Geometry: final body of the model. Coordinates: model frame, mm. Face numbers are marked on the shaded views. A direction names the side the tool comes from. Give positions to 0.01 mm unless a question says otherwise; leave off trailing zeros. Write each loop counter-clockwise with the first axis right and the second up, starting at its lowest first coordinate (ties: lowest second). Pieces come first, ordered by that corner, then holes. Notation, with made-up numbers: M -39.75,-30 L -5.75,-30 A17 ccw -5.75,-2 Z; hole C 7.25,-29 d3. An arc over 180 degrees is marked long. Use one line per item in the form item = value. Start each with the question number.
Item 1: Access query for the marked faces 1 and 2. Directions: +Z, -Z, +X, -X, +Y, -Y. A direction counts if a zero-diameter tool reaches every point of the face in a straight line with its end or side. Return the directions, or none.
Item 2: Material intervals for line 1 along X through (y, z) = (-7.5, 1.05); line 2 along X through (y, z) = (-15.5, 2.2); line 3 along Y through (x, z) = (-57.5, 1.65), sorted ascending. Write a range as from..to.
Item 3: Section query A-A on y = 8. Return loops of the section in (x, z), then the cut area to 3 significant figures.
Item 4: Pull-direction query (Y, two-part tool) for the marked faces 3, 4 and 5; classes: released by +Y, released by -Y, zero draft, split by the parting line, or undercut.
Item 5: Section query B-B on x = -43. Return loops of the section in (y, z).
Item 6: Section query C-C on y = 1.5. Return loops of the section in (x, z), then the cut area to 3 significant figures.
Item 7: Contact query for a flat-ended pin moving along its axis: P1, Ø2, axis at x = -57.5, y = -7.5, coming from the +Z side. Output: stop coordinate, or through.
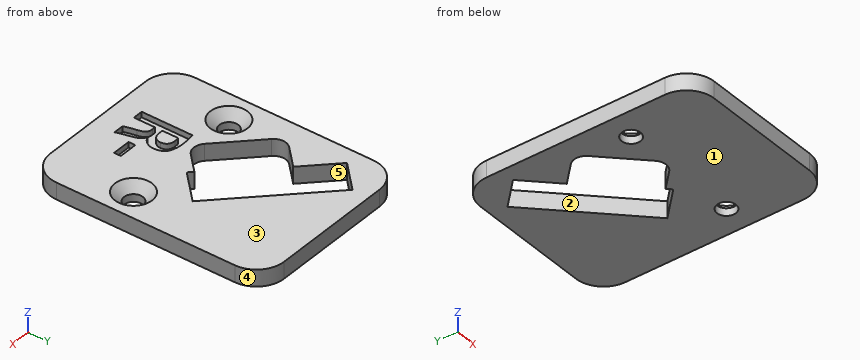
from build123d import *

# Parameters (mm, degrees)
SKETCH2_W                                           = 32
SKETCH2_H                                           = 42.204432033
BOSS_EXTRUDE2_DEPTH                                 = 3
FILLET1_R                                           = 5
SKETCH3_W                                           = 3.336226562
SKETCH3_H                                           = 1.222113554
CUT_EXTRUDE1_DEPTH                                  = 1
CSK_FOR_M3_COUNTERSUNK_FLAT_HEAD_SCREW1_D           = 3.4
CSK_FOR_M3_COUNTERSUNK_FLAT_HEAD_SCREW1_DEPTH       = 20
CSK_FOR_M3_COUNTERSUNK_FLAT_HEAD_SCREW1_CSINK_D     = 6.7
CSK_FOR_M3_COUNTERSUNK_FLAT_HEAD_SCREW1_CSINK_ANGLE = 90
CSK_FOR_M3_COUNTERSUNK_FLAT_HEAD_SCREW1_TIP         = 1.021463052
CUT_EXTRUDE3_DEPTH                                  = 10


with BuildPart() as part:
    # Sketch2 → Boss-Extrude2 (new body)
    with BuildSketch(Plane.XY):
        with Locations((-46.5, -1.397783984)):
            Rectangle(SKETCH2_W, SKETCH2_H)
    extrude(amount=BOSS_EXTRUDE2_DEPTH)

    # Fillet1
    fillet1_edges = [part.edges().sort_by_distance(p)[0] for p in [
        (-62.5, 19.704432033, 1.5),
        (-30.5, 19.704432033, 1.5),
        (-30.5, -22.5, 1.5),
        (-62.5, -22.5, 1.5),
    ]]
    fillet(fillet1_edges, radius=FILLET1_R)

    # Sketch3 → Cut-Extrude1 (cut)
    with BuildSketch(Plane.XY.offset(3)):
        with BuildLine():
            Line((-51.381425439, -18.458875061), (-49.597421385, -18.458875061))
            Line((-49.597421385, -18.458875061), (-49.597421385, -14.672122679))
            Line((-49.597421385, -14.672122679), (-48.991938415, -14.672122679))
            add(Edge.make_bspline(
                [(-48.991938415, -14.672122679), (-48.942050564, -14.6725211), (-48.843919084, -14.673304811), (-48.701136712, -14.687536776), (-48.566178681, -14.711269605), (-48.441222715, -14.74890661), (-48.32427753, -14.795186794), (-48.218202264, -14.856795477), (-48.11890245, -14.926037335), (-48.029787183, -15.010644116), (-47.94865002, -15.109304476), (-47.870329282, -15.22163632), (-47.801359571, -15.353586411), (-47.734046558, -15.500135947), (-47.675917518, -15.664809001), (-47.618382932, -15.843956856), (-47.570508607, -16.041536599), (-47.542007813, -16.179191645), (-47.527206071, -16.25068209)],
                knots=[0, 0, 0, 0, 0.000149599, 0.000294267, 0.000429961, 0.000559969, 0.000685182, 0.000806276, 0.000927115, 0.001047609, 0.001173509, 0.001309883, 0.001457588, 0.001619475, 0.001793345, 0.001981055, 0.002183769, 0.002402801, 0.002402801, 0.002402801, 0.002402801], degree=3))
            add(Edge.make_bspline(
                [(-47.527206071, -16.25068209), (-47.500027556, -16.387123246), (-47.447932519, -16.648649934), (-47.367799698, -17.023584407), (-47.286395279, -17.362673147), (-47.211369572, -17.666100231), (-47.134583702, -17.927379781), (-47.069987521, -18.146751884), (-47.009849282, -18.32008565), (-46.966417008, -18.417682148), (-46.947756493, -18.45961412)],
                knots=[0, 0, 0, 0, 0.000417367, 0.000799998, 0.001150089, 0.001463532, 0.001737527, 0.001966934, 0.002149658, 0.002287303, 0.002287303, 0.002287303, 0.002287303], degree=3))
            Line((-46.947756493, -18.45961412), (-45.111733669, -18.458875061))
            add(Edge.make_bspline(
                [(-45.111733669, -18.458875061), (-45.136394395, -18.402686862), (-45.192836553, -18.274086301), (-45.264632108, -18.048232695), (-45.345858267, -17.770288113), (-45.428958388, -17.444111213), (-45.51591734, -17.08294144), (-45.610026609, -16.699954349), (-45.704155867, -16.299301278), (-45.768362179, -16.026508782), (-45.80114869, -15.887209172)],
                knots=[0, 0, 0, 0, 0.000183977, 0.000421076, 0.000710029, 0.001052867, 0.00143062, 0.001824558, 0.002235981, 0.002665299, 0.002665299, 0.002665299, 0.002665299], degree=3))
            add(Edge.make_bspline(
                [(-45.80114869, -15.887209172), (-45.828641018, -15.773168942), (-45.881780404, -15.5527428), (-45.987295673, -15.242137194), (-46.108403792, -14.961961493), (-46.246109756, -14.712628496), (-46.405457942, -14.494327391), (-46.588613385, -14.309294243), (-46.799272936, -14.160659908), (-46.954100619, -14.089741414), (-47.032040068, -14.054041414)],
                knots=[0, 0, 0, 0, 0.000351778, 0.000679945, 0.00098268, 0.001266475, 0.001532679, 0.001790935, 0.002044255, 0.002301038, 0.002301038, 0.002301038, 0.002301038], degree=3))
            Line((-47.032040068, -14.054041414), (-47.030656262, -14.017001018))
            add(Edge.make_bspline(
                [(-47.030656262, -14.017001018), (-46.922273974, -13.970005767), (-46.706005829, -13.876230519), (-46.411856808, -13.676157256), (-46.14181559, -13.438863882), (-45.942211161, -13.208200023), (-45.802357006, -13.003332314), (-45.709339658, -12.840203194), (-45.629535439, -12.668874791), (-45.565066724, -12.488727388), (-45.51180506, -12.300576236), (-45.473637881, -12.103222096), (-45.448546386, -11.89781805), (-45.443663093, -11.757970901), (-45.441187588, -11.68707768)],
                knots=[0, 0, 0, 0, 0.000353722, 0.000705825, 0.001061629, 0.00143016, 0.001617179, 0.001805135, 0.001992894, 0.002183416, 0.002378543, 0.002578963, 0.00278587, 0.002998596, 0.002998596, 0.002998596, 0.002998596], degree=3))
            add(Edge.make_bspline(
                [(-45.441187588, -11.68707768), (-45.446164978, -11.614412673), (-45.455946444, -11.471612893), (-45.485146081, -11.263842973), (-45.519750271, -11.065622921), (-45.563079094, -10.87842638), (-45.616257063, -10.701449), (-45.677340843, -10.534699828), (-45.747075442, -10.378252437), (-45.826987856, -10.232984263), (-45.914816466, -10.098344998), (-46.008796832, -9.971834439), (-46.116049062, -9.860313263), (-46.228017531, -9.754798011), (-46.351436153, -9.662838486), (-46.482253648, -9.578828028), (-46.62263241, -9.507518301), (-46.818699815, -9.427166253), (-47.06746288, -9.344888092), (-47.360362202, -9.252977107), (-47.648888658, -9.184061361), (-47.928465046, -9.126227189), (-48.201942503, -9.088865813), (-48.467771392, -9.061958609), (-48.727193986, -9.057551627), (-48.897426641, -9.065240143), (-48.981097742, -9.069019128)],
                knots=[0, 0, 0, 0, 0.000218439, 0.000429273, 0.000629045, 0.000821988, 0.00100531, 0.001183082, 0.001354416, 0.001518656, 0.001679866, 0.001836496, 0.001990536, 0.002143381, 0.002297551, 0.002451481, 0.002609328, 0.002769115, 0.003086745, 0.003395031, 0.003689736, 0.003976245, 0.004251139, 0.004517418, 0.004777346, 0.005028594, 0.005028594, 0.005028594, 0.005028594], degree=3))
            add(Edge.make_bspline(
                [(-48.981097742, -9.069019128), (-49.204750164, -9.07164849), (-49.641894612, -9.076787763), (-50.178628932, -9.112050461), (-50.585677154, -9.150113546), (-50.867868242, -9.181499683), (-51.131979771, -9.216172913), (-51.301297073, -9.243625216), (-51.383179632, -9.256901264)],
                knots=[0, 0, 0, 0, 0.000670904, 0.001311329, 0.001612901, 0.001897363, 0.00216308, 0.002411924, 0.002411924, 0.002411924, 0.002411924], degree=3))
            Line((-51.383179632, -9.256901264), (-51.381425439, -18.458875061))
        make_face()
        with BuildLine():
            add(Edge.make_bspline(
                [(-49.597421385, -10.475098321), (-49.553118884, -10.463741178), (-49.449324767, -10.437133094), (-49.26651153, -10.418528414), (-49.036966225, -10.403821129), (-48.868179272, -10.40361956), (-48.775656528, -10.403509067)],
                knots=[0, 0, 0, 0, 0.000137048, 0.000321084, 0.000549784, 0.00082724, 0.00082724, 0.00082724, 0.00082724], degree=3))
            add(Edge.make_bspline(
                [(-48.775656528, -10.403509067), (-48.688241346, -10.402981113), (-48.513173263, -10.40192377), (-48.25262374, -10.452443011), (-47.99710085, -10.54015698), (-47.790180436, -10.642172207), (-47.635138174, -10.749873331), (-47.531709547, -10.851803167), (-47.444125211, -10.972739958), (-47.368662464, -11.111515899), (-47.313363495, -11.270485036), (-47.266241854, -11.445599811), (-47.237372321, -11.640002112), (-47.229365771, -11.775957367), (-47.225189927, -11.846865291)],
                knots=[0, 0, 0, 0, 0.000261725, 0.000524161, 0.000791249, 0.001070808, 0.00121308, 0.001355871, 0.001504077, 0.001659631, 0.001827951, 0.00200768, 0.002203123, 0.002416175, 0.002416175, 0.002416175, 0.002416175], degree=3))
            add(Edge.make_bspline(
                [(-47.225189927, -11.846865291), (-47.227175329, -11.901954186), (-47.231054857, -12.009599393), (-47.252578328, -12.166460507), (-47.285644456, -12.315396112), (-47.332465946, -12.455901219), (-47.395176387, -12.587424294), (-47.470077536, -12.710240218), (-47.559607688, -12.823418468), (-47.659086339, -12.929228854), (-47.771771397, -13.023790308), (-47.894893734, -13.107175482), (-48.0305682, -13.175598565), (-48.175685207, -13.233265514), (-48.331962757, -13.279426838), (-48.49835821, -13.311908188), (-48.675604243, -13.333661231), (-48.79724634, -13.337439587), (-48.859940103, -13.339386933)],
                knots=[0, 0, 0, 0, 0.000165289, 0.000322979, 0.000474201, 0.000622458, 0.000766196, 0.000910448, 0.001053055, 0.001198372, 0.001345408, 0.001493457, 0.001643451, 0.001800288, 0.001961411, 0.002131526, 0.002308376, 0.002496463, 0.002496463, 0.002496463, 0.002496463], degree=3))
            Line((-48.859940103, -13.339386933), (-49.597421385, -13.33763274))
            Line((-49.597421385, -13.33763274), (-49.597421385, -10.475098321))
        make_face(mode=Mode.SUBTRACT)
        with Locations((-42.847712603, -14.847712603)):
            Rectangle(SKETCH3_W, SKETCH3_H)
    extrude(amount=-CUT_EXTRUDE1_DEPTH, mode=Mode.SUBTRACT)

    # CSK for M3 Countersunk Flat Head Screw1
    with Locations(Plane(origin=(-57.5, -7.5, 3), x_dir=(1, 0, 0), z_dir=(0, 0, 1))):
        with Locations((0, 0), (22, 0)):
            CounterSinkHole(CSK_FOR_M3_COUNTERSUNK_FLAT_HEAD_SCREW1_D / 2, CSK_FOR_M3_COUNTERSUNK_FLAT_HEAD_SCREW1_CSINK_D / 2, depth=CSK_FOR_M3_COUNTERSUNK_FLAT_HEAD_SCREW1_DEPTH, counter_sink_angle=CSK_FOR_M3_COUNTERSUNK_FLAT_HEAD_SCREW1_CSINK_ANGLE)
            with Locations((0, 0, -(CSK_FOR_M3_COUNTERSUNK_FLAT_HEAD_SCREW1_DEPTH + CSK_FOR_M3_COUNTERSUNK_FLAT_HEAD_SCREW1_TIP / 2))):  # 118° drill point
                Cone(0, CSK_FOR_M3_COUNTERSUNK_FLAT_HEAD_SCREW1_D / 2, CSK_FOR_M3_COUNTERSUNK_FLAT_HEAD_SCREW1_TIP, mode=Mode.SUBTRACT)

    # Sketch13 → Cut-Extrude3 (cut)
    with BuildSketch(Plane(origin=(0, 0, 0), x_dir=(-1, 0, 0), z_dir=(0, 0, -1))):
        with BuildLine():
            Line((55.099076528, 16.704432033), (59.695270606, 12.108237955))
            Line((59.695270606, 12.108237955), (54.250548391, 6.66351574))
            Line((54.250548391, 6.66351574), (57.609305602, 3.304758529))
            ThreePointArc((57.609305602, 3.304758529), (58.268315344, 1.713768272), (57.609305602, 0.122778014))
            Line((57.609305602, 0.122778014), (50.821080502, -6.665447085))
            ThreePointArc((50.821080502, -6.665447085), (49.230090245, -7.324456828), (47.639099987, -6.665447085))
            Line((47.639099987, -6.665447085), (44.633896167, -3.660243265))
            Line((44.633896167, -3.660243265), (43.856078708, -4.438060725))
            Line((43.856078708, -4.438060725), (43.325748622, -3.907730639))
            Line((43.325748622, -3.907730639), (38.906331239, 0.511686744))
            Line((38.906331239, 0.511686744), (40.709453531, 2.314809036))
            Line((40.709453531, 2.314809036), (47.921942699, 9.527298204))
            Line((47.921942699, 9.527298204), (55.099076528, 16.704432033))
        make_face()
    extrude(amount=-CUT_EXTRUDE3_DEPTH, mode=Mode.SUBTRACT)


solid = part.part
Answer sheet:
q1.face_1 = -Z, +X, -X, +Y, -Y
q1.face_2 = +Z, -Z
q2.line_1 = -62.5..-59.2, -55.8..-37.2, -33.8..-30.5
q2.line_2 = -62.5..-51.38, -49.6..-47.74, -45.9..-30.5
q2.line_3 = -22.5..-9.5, -5.5..0.01, 3.41..9.91, 14.3..19.7
q3.outline = M -62.5,0 L -55.59,0 L -55.59,3 L -62.5,3 Z; M -46.39,0 L -30.5,0 L -30.5,3 L -46.39,3 Z
q3.area = 68.4 mm2
q4.face_3 = zero draft
q4.face_4 = released by +Y
q4.face_5 = undercut
q5.outline = M -22.5,0 L -3.58,0 L -3.58,3 L -14.24,3 L -14.24,2 L -15.46,2 L -15.46,3 L -22.5,3 Z; M 4.61,0 L 19.7,0 L 19.7,3 L 4.61,3 Z
q6.outline = M -62.5,0 L -58.26,0 L -58.26,3 L -62.5,3 Z; M -39.89,0 L -30.5,0 L -30.5,3 L -39.89,3 Z
q6.area = 40.9 mm2
q7.P1 = through
